Model file for the job. Use its own axes, mm. A direction names the side the tool comes from. Give positions to 0.01 mm unless a question says otherwise; leave off trailing zeros. Write each loop counter-clockwise with the first axis right and the second up, starting at its lowest first coordinate (ties: lowest second). Pieces come first, ordered by that corner, then holes.
```python
from build123d import *

# Parameters (mm, degrees)
SALIENTE_EXTRUIR1_DEPTH = 15
CROQUIS3_R              = 3.5
SALIENTE_EXTRUIR2_DEPTH = 6
CROQUIS5_R              = 2
SALIENTE_EXTRUIR4_DEPTH = 2
CROQUIS7_R              = 3.5
SALIENTE_EXTRUIR5_DEPTH = 2


with BuildPart() as part:
    # Croquis2 → Saliente-Extruir1 (new body)
    with BuildSketch(Plane(origin=(0, 0, 0), x_dir=(1, 0, 0), z_dir=(0, 1, 0))):
        with BuildLine():
            Line((0, 10), (0, -10))
            ThreePointArc((0, -10), (-10, 0), (0, 10))
        make_face()
    extrude(amount=SALIENTE_EXTRUIR1_DEPTH)

    # Croquis3 → Saliente-Extruir2 (add)
    with BuildSketch(Plane.XZ):
        with Locations(Location((-5, 0, 0), (0, 0, 270))):
            Circle(CROQUIS3_R)
    extrude(amount=SALIENTE_EXTRUIR2_DEPTH)

    # Croquis5 → Saliente-Extruir4 (add)
    with BuildSketch(Plane.XZ.offset(6)):
        with Locations(Location((-5, 0, 0), (0, 0, 270))):
            Circle(CROQUIS5_R)
    extrude(amount=SALIENTE_EXTRUIR4_DEPTH)

    # Croquis7 → Saliente-Extruir5 (add)
    with BuildSketch(Plane.XZ.offset(8)):
        with Locations(Location((-5, 0, 0), (0, 0, 270))):
            Circle(CROQUIS7_R)
    extrude(amount=SALIENTE_EXTRUIR5_DEPTH)


solid = part.part
```
1. Slice it at D-D, the plane z = 4.25. Write the cut outline in (x, y).
Calculated:
outline: (-9.05, 0) - (0, 0) - (0, 15) - (-9.05, 15) - close
2. Slice it at A-A, the plane z = 0. Write the cut outline in (x, y), and give its area (3 significant figures).
Calculated:
outline: (-10, 0) - (-8.5, 0) - (-8.5, -6) - (-7, -6) - (-7, -8) - (-8.5, -8) - (-8.5, -10) - (-1.5, -10) - (-1.5, -8) - (-3, -8) - (-3, -6) - (-1.5, -6) - (-1.5, 0) - (0, 0) - (0, 15) - (-10, 15) - close
area: 214 mm2
3. Slice it at C-C, the plane y = 4.5. Write the cut outline in (x, z), and give its area (3 significant figures).
Calculated:
outline: (0, -10) - (0, 10) arc R10 ccw to start
area: 157 mm2
4. Slice it at B-B, the plane x = -5. Write the cut outline in (y, z), and give its area (3 significant figures).
Calculated:
outline: (-10, -3.5) - (-8, -3.5) - (-8, -2) - (-6, -2) - (-6, -3.5) - (0, -3.5) - (0, -8.66) - (15, -8.66) - (15, 8.66) - (0, 8.66) - (0, 3.5) - (-6, 3.5) - (-6, 2) - (-8, 2) - (-8, 3.5) - (-10, 3.5) - close
area: 324 mm2
5. Pull direction Y, two halves, no side cores. Call faces 4 (the cylindrical face through (-8.417, -8.986, 0.759)), 5 (the flat face through (-7, -8, -2)), 6 (the flat face through (-5, -10, 0)): +Y half, -Y half, draft (parallel to the pull), parting line (faces both ways), or undercut.
Calculated:
face 4: draft
face 5: undercut
face 6: -Y half
6. Which spindle directions (+Z, -Z, +X, -X, +Y, -Y) get a long thin tool onto all of the face, cutting with end or side? Do faces 1 (the flat face through (-4, 15, 0)), 2 (the cylindrical face through (-7, -7, 0)), 3 (the cylindrical face through (-8.417, -2.958, 0.759)). Say none if no direction does.
Calculated:
face 1: +Z, -Z, +X, -X, +Y
face 2: none
face 3: -Y
7. Pin check, flat tips, straight feed: P1, Ø4, axis at y = -5.5, z = 0, coming from the +X side; P2, Ø10, axis at y = -0.5, z = 4, coming from the +X side; P3, Ø3, axis at x = -4, z = -5.5, coming from the -Y side. Stop position of each tip, or through.
Calculated:
P1: stops at x = -1.5
P2: stops at x = 0
P3: stops at y = 0
8. Probe probe 1 along Y at (x, z) = (-7.25, -2.25); probe 2 along Y at (x, z) = (-3.5, 7); probe 3 along X at (y, z) = (2.25, 0). List the from-to ranges inside material, lowest first.
Calculated:
probe 1: y = -10 to -8, -6 to 15
probe 2: y = 0 to 15
probe 3: x = -10 to 0
